from build123d import *

# Parameters (mm, degrees)
EXTRUDE_1_DEPTH     = 3
SKETCH_2_W          = 5
SKETCH_2_H          = 3
CUT_EXTRUDE_1_DEPTH = 176
SKETCH_3_W          = 146.2
SKETCH_3_H          = 3
EXTRUDE_2_DEPTH     = 5
SKETCH_4_R          = 1.7
CUT_EXTRUDE_2_DEPTH = 5
CUT_EXTRUDE_3_DEPTH = 10
FILLET_1_R          = 5
FILLET_2_R          = 5


with BuildPart() as part:
    # 草图1 → 凸台-拉伸1 (new body)
    with BuildSketch(Plane(origin=(0, 0, 0), x_dir=(1, 0, 0), z_dir=(0, 1, 0))):
        Polygon((-25, -73.1), (-25, -76.1), (-20, -76.1), (-20, -73.1), (-13.7, -73.1), (-13.7, -68.1), (-15.4, -68.1), (-15.4, -65.1), (-13.7, -65.1), (-13.7, -60.1), (-10.3, -60.1), (-10.3, -65.1), (-8.6, -65.1), (-8.6, -68.1), (-10.3, -68.1), (-10.3, -73.1), (-4, -73.1), (-4, -76.1), (4, -76.1), (4, -73.1), (10.3, -73.1), (10.3, -68.1), (8.6, -68.1), (8.6, -65.1), (10.3, -65.1), (10.3, -60.1), (13.7, -60.1), (13.7, -65.1), (15.4, -65.1), (15.4, -68.1), (13.7, -68.1), (13.7, -73.1), (20, -73.1), (20, -76.1), (25, -76.1), (25, -73.1), (35, -73.1), (35, 73.1), (25, 73.1), (25, 76.1), (20, 76.1), (20, 73.1), (13.7, 73.1), (13.7, 68.1), (15.4, 68.1), (15.4, 65.1), (13.7, 65.1), (13.7, 60.1), (10.3, 60.1), (10.3, 65.1), (8.6, 65.1), (8.6, 68.1), (10.3, 68.1), (10.3, 73.1), (4, 73.1), (4, 76.1), (-4, 76.1), (-4, 73.1), (-10.3, 73.1), (-10.3, 68.1), (-8.6, 68.1), (-8.6, 65.1), (-10.3, 65.1), (-10.3, 60.1), (-13.7, 60.1), (-13.7, 65.1), (-15.4, 65.1), (-15.4, 68.1), (-13.7, 68.1), (-13.7, 73.1), (-20, 73.1), (-20, 76.1), (-25, 76.1), (-25, 73.1), (-35, 73.1), (-35, -73.1), align=None)
    extrude(amount=EXTRUDE_1_DEPTH)

    # 草图2 → 切除-拉伸1 (cut)
    with BuildSketch(Plane.XY.offset(73.1)):
        with Locations((-32.5, 1.5)):
            Rectangle(SKETCH_2_W, SKETCH_2_H)
    extrude(amount=-CUT_EXTRUDE_1_DEPTH, mode=Mode.SUBTRACT)

    # 草图3 → 凸台-拉伸2 (add)
    with BuildSketch(Plane(origin=(35, 0, 0), x_dir=(0, 0, -1), z_dir=(1, 0, 0))):
        with Locations((0, 1.5)):
            Rectangle(SKETCH_3_W, SKETCH_3_H)
    extrude(amount=EXTRUDE_2_DEPTH)

    # 草图4 → 切除-拉伸2 (cut)
    with BuildSketch(Plane(origin=(0, 3, 0), x_dir=(1, 0, 0), z_dir=(0, 1, 0))):
        with Locations(Location((-19.75, -58.1, 0), (0, 0, 270))):
            Circle(SKETCH_4_R)
        with Locations(Location((19.25, -58.1, 0), (0, 0, 270))):
            Circle(SKETCH_4_R)
        with Locations(Location((19.25, 58.1, 0), (0, 0, 270))):
            Circle(SKETCH_4_R)
        with Locations(Location((-19.75, 58.1, 0), (0, 0, 270))):
            Circle(SKETCH_4_R)
    extrude(amount=-CUT_EXTRUDE_2_DEPTH, mode=Mode.SUBTRACT)

    # 草图5 → 切除-拉伸3 (cut)
    with BuildSketch(Plane(origin=(0, 3, 0), x_dir=(1, 0, 0), z_dir=(0, 1, 0))):
        Polygon((-30, -56.331395183), (-14.5, -43.1), (0, -43.1), (22, -43.1), (22, 43.1), (-14.5, 43.1), (-30, 56.331395183), align=None)
    extrude(amount=-CUT_EXTRUDE_3_DEPTH, mode=Mode.SUBTRACT)

    # 圆角1
    fillet_1_edges = [part.edges().sort_by_distance(p)[0] for p in [
        (-30, 1.5, 56.331395183),
        (-30, 1.5, -56.331395183),
        (-14.5, 1.5, -43.1),
        (22, 1.5, -43.1),
        (22, 1.5, 43.1),
        (-14.5, 1.5, 43.1),
    ]]
    fillet(fillet_1_edges, radius=FILLET_1_R)

    # 圆角2
    fillet_2_edges = [part.edges().sort_by_distance(p)[0] for p in [
        (40, 1.5, 73.1),
        (40, 1.5, -73.1),
    ]]
    fillet(fillet_2_edges, radius=FILLET_2_R)


solid = part.part
Geometry: final body of the model. Coordinates: model frame, mm. A direction names the side the tool comes from. Give positions to 0.01 mm unless a question says otherwise; leave off trailing zeros. Order: outer loops, then holes, each group sorted by start corner. A loop starts at its lowest first (then second) coordinate and runs counter-clockwise, first axis right, second up. Notation, with made-up numbers: (78.25, -24) -> (135.25, -24) arc R20 ccw to (135.25, 14) -> close; hole circle Ø9 at (-37.75, -2). An arc over 180 degrees is marked (long way). Answer as a JSON object with one key per item and string values.
Q1. Section B-B (y = 1.65). State how many separate pieces and enclosed holes the cut face has, plus the area to 3 significant figures.
Entries:
{"separate pieces": "1", "enclosed holes": "4", "area": "5,400 mm^2"}
Q2. Draft query along X for faces 1 (the flat face through (-10.3, 1, 63)), 2 (the cylindrical face through (38.57, 1.52, -71.6)), 3 (the flat face through (-30, 1, -66)). Return one class per face: released by +X, released by -X, zero draft, split by the parting line, or undercut.
Entries:
{"face 1": "undercut", "face 2": "released by +X", "face 3": "released by -X"}
Q3. Section C-C (x = 27). Output: boundary loops of the cut face in (y, z), plus the area to 3 significant figures.
Entries:
{"outline": "(0, -73.1) -> (3, -73.1) -> (3, 73.1) -> (0, 73.1) -> close", "area": "439 mm^2"}
Q4. Material intervals for probe 1 along X at (y, z) = (2.05, 58.1); probe 2 along X at (y, z) = (0.55, 62); probe 3 along Z at (x, y) = (14, 1.1), sorted ascending.
Entries:
{"probe 1": "x = -29.97 to -21.45, -18.05 to 17.55, 20.95 to 40", "probe 2": "x = -30 to -13.7, -10.3 to 10.3, 13.7 to 40", "probe 3": "z = -73.1 to -68.1, -65.1 to -43.1, 43.1 to 65.1, 68.1 to 73.1"}
Q5. Section A-A (z = 33). Output: boundary loops of the cut face in (x, y), plus the area to 3 significant figures.
Entries:
{"outline": "(22, 0) -> (40, 0) -> (40, 3) -> (22, 3) -> close", "area": "54.0 mm^2"}
Q6. Access query for faces 4 (the flat face through (-10.3, 1, -63)), 5 (the flat face through (13.7, 1, 71)), 6 (the flat face through (-15.4, 1, -67)), 7 (the flat face through (2, 2, 43.1)). Directions: +Z, -Z, +X, -X, +Y, -Y. A direction counts if a zero-diameter tool reaches every point of the face in a straight line with its end or side. Return the directions, or none.
Entries:
{"face 4": "-Z, +Y, -Y", "face 5": "+Z, +Y, -Y", "face 6": "+Y, -Y", "face 7": "-X, +Y, -Y"}
Q7. First-contact query: pin 1 (4 mm diameter, centred on x = 29.5, z = 57.5, fed in from -Y); pin 2 (1.5 mm diameter, centred on x = -7.5, y = 1.5, fed in from -Z); pin 3 (1.5 mm diameter, centred on y = 2, z = -74.5, fed in from -X). Flat tips, straight axial feed; report the tip coordinate or a pass-through.
Entries:
{"pin 1": "stops at y = 0", "pin 2": "stops at z = -73.1", "pin 3": "stops at x = -25"}
